Geometry check sheet. Reference: drawing and pictorial views, mm from the part's lowest x, y, z. Give positions to 0.01 mm unless a question says otherwise; leave off trailing zeros. Loops run counter-clockwise (first coordinate to the right, second up) from the corner with the lowest first, then second, coordinate; pieces in that order, holes last. Notation, with made-up numbers: M -29,1.25 L 7,1.25 A24 ccw 7,33.25 Z; hole C 87,2 d7. An arc over 180 degrees is marked long. Use CSV: the item, a comma, the result in double quotes.
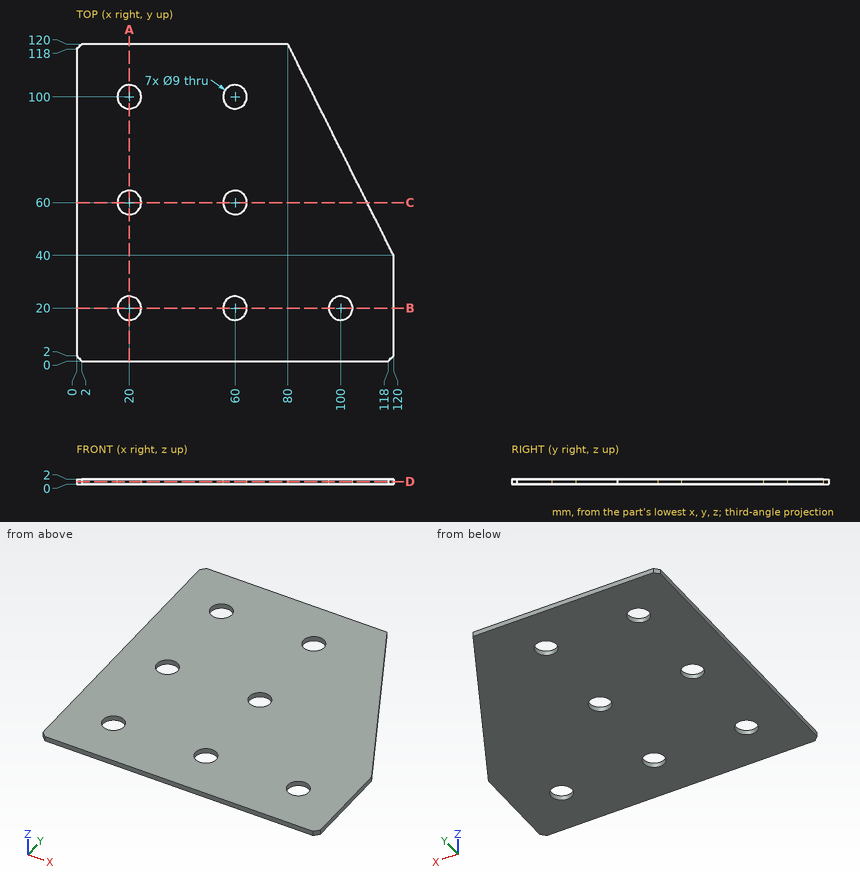
(1) Section check A-A on x = 20. Record the cut outline in (y, z), plus the area to 3 significant figures.
Calculated:
outline,"M 0,0 L 15.5,0 L 15.5,2 L 0,2 Z; M 24.5,0 L 55.5,0 L 55.5,2 L 24.5,2 Z; M 64.5,0 L 95.5,0 L 95.5,2 L 64.5,2 Z; M 104.5,0 L 120,0 L 120,2 L 104.5,2 Z"
area,"186 mm²"
(2) Depth check by flat-ended pin: pin 1 Ø11.5 at (x, y) = (100, 20) entering from -Z; pin 2 Ø2 at (x, y) = (58, 57.5) entering from +Z. Enter the tip coordinate at first touch or a pass-through.
Calculated:
pin 1,"stops at z = 0"
pin 2,"passes through"
(3) Section check D-D on z = 1. Record the cut outline in (x, y).
Calculated:
outline,"M 0,2 L 2,0 L 118,0 L 120,2 L 120,40 L 80,120 L 2,120 L 0,118 Z; hole C 20,20 d9; hole C 20,60 d9; hole C 20,100 d9; hole C 60,20 d9; hole C 60,60 d9; hole C 60,100 d9; hole C 100,20 d9"
(4) Scan lines: L1, parallel to Y at x = 20, z = 1.4; L2, parallel to Y at x = 100, z = 0.7. Record each from-to range of solid material in increasing order. Write a range as from..to.
Calculated:
L1,"y = 0..15.5, 24.5..55.5, 64.5..95.5, 104.5..120"
L2,"y = 0..15.5, 24.5..80"
(5) Section check C-C on y = 60. Record the cut outline in (x, z).
Calculated:
outline,"M 0,0 L 15.5,0 L 15.5,2 L 0,2 Z; M 24.5,0 L 55.5,0 L 55.5,2 L 24.5,2 Z; M 64.5,0 L 110,0 L 110,2 L 64.5,2 Z"
